Part print with two shaded views. Sizes in mm from the minimum x, y, z corner. A direction names the side the tool comes from. Round coordinates to 2 decimals unless told otherwise and drop trailing zeros. Write each loop counter-clockwise with the first axis right and the second up, starting at its lowest first coordinate (ties: lowest second). Pieces come first, ordered by that corner, then holes. Notation, with made-up numbers: M 33,16 L 87,16 A12 cw 87,30 Z; hole C 84,26.25 d10. An arc over 180 degrees is marked long. Use one line per item in the form item = value. Start each with the question number.
Item 1: Flat gauge pins, fed straight in: pin 1 Ø1 at (x, y) = (15, 19) entering from +Z; pin 2 Ø6.5 at (y, z) = (59.5, 35) entering from -X; pin 3 Ø2.5 at (x, y) = (11, 5) entering from +Z. Where does each tip first touch, or does it go through?
Item 2: Which spindle directions (+Z, -Z, +X, -X, +Y, -Y) get a long thin tool onto all of the face, cutting with end or side? Do the marked faces 4, 5 and 6. Say none if no direction does.
Item 3: Cut at C-C, the plane x = 14.75. Give the cut face in (y, z), then the cut area to 3 significant figures.
Item 4: Probe L1, parallel to Y at x = 25.25, z = 32.5; L2, parallel to Y at x = 21, z = 27; L3, parallel to Z at x = 21.5, y = 38. List the from-to ranges inside material, lowest first.
Item 5: Cut at D-D, the plane x = 9.25. Give the cut face in (y, z).
Item 6: Cut at A-A, the plane y = 31.5. Give the cut face in (x, z), then the cut area to 3 significant figures.
Item 7: Mould opens along Y. For the marked faces 1, 2 and 3 say: +Y half, -Y half, draft (parallel to the pull), parting line (faces both ways), or undercut.
Item 8: Cut at B-B, the plane z = 22.5. Give the cut face in (x, y), then the cut area to 4 significant figures.
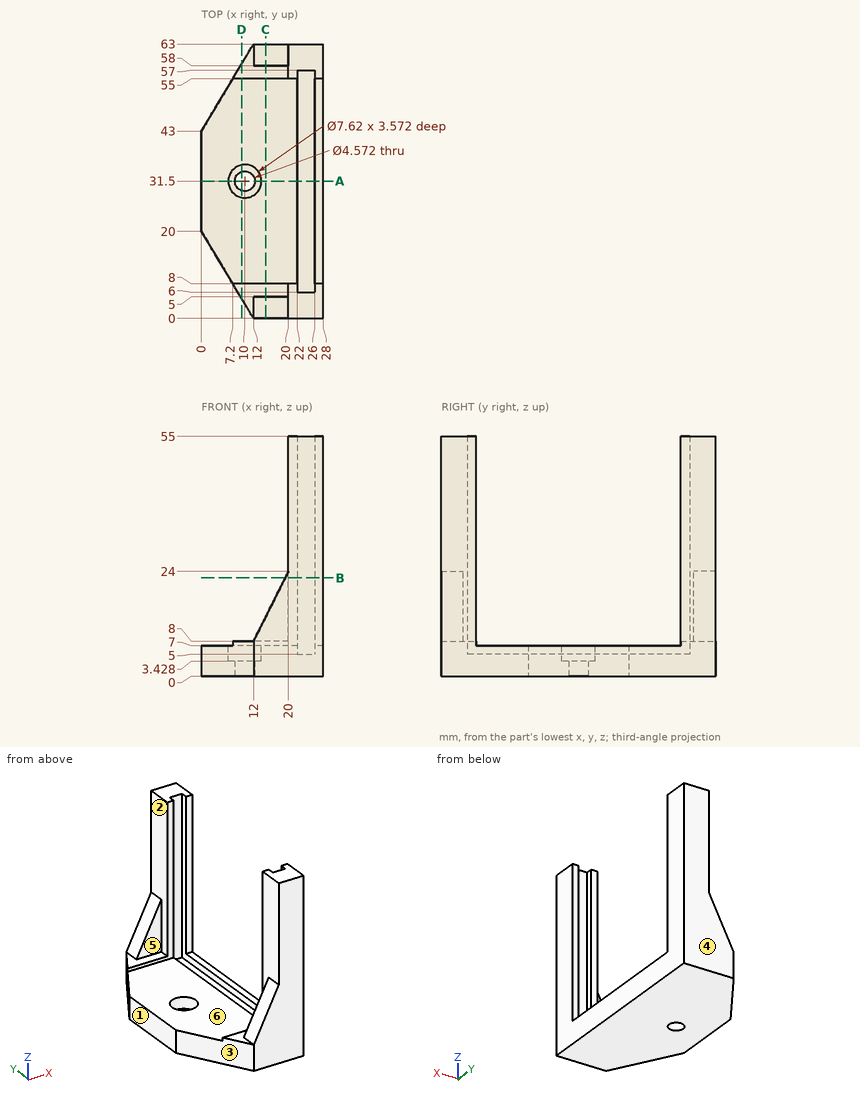
Model answer:
q1.pin_1 = 7
q1.pin_2 = 20
q1.pin_3 = 8.5
q2.face_4 = +Z, -Z, +X, -X, +Y
q2.face_5 = +Z, -X
q2.face_6 = +Z, +X, -X
q3.outline = M 0,0 L 63,0 L 63,13.5 L 58,13.5 L 58,8 L 55,8 L 55,7 L 8,7 L 8,8 L 5,8 L 5,13.5 L 0,13.5 Z
q3.area = 512 mm²
q4.L1 = 0 to 6, 57 to 63
q4.L2 = 0 to 8, 55 to 63
q4.L3 = 0 to 7
q5.outline = M 4.58,0 L 29.34,0 L 29.34,3.43 L 27.76,3.43 L 27.76,7 L 8,7 L 8,8 L 4.58,8 Z; M 33.66,0 L 58.42,0 L 58.42,8 L 55,8 L 55,7 L 35.24,7 L 35.24,3.43 L 33.66,3.43 Z
q6.outline = M 0,0 L 7.71,0 L 7.71,3.43 L 6.19,3.43 L 6.19,7 L 0,7 Z; M 12.29,0 L 28,0 L 28,7 L 26,7 L 26,5 L 22,5 L 22,7 L 13.81,7 L 13.81,3.43 L 12.29,3.43 Z
q6.area = 145 mm²
q7.face_1 = draft
q7.face_2 = undercut
q7.face_3 = -Y half
q8.outline = M 19.25,0 L 28,0 L 28,8 L 26,8 L 26,6 L 22,6 L 22,8 L 20,8 L 20,5 L 19.25,5 Z; M 19.25,58 L 20,58 L 20,55 L 22,55 L 22,57 L 26,57 L 26,55 L 28,55 L 28,63 L 19.25,63 Z
q8.area = 119.5 mm²
